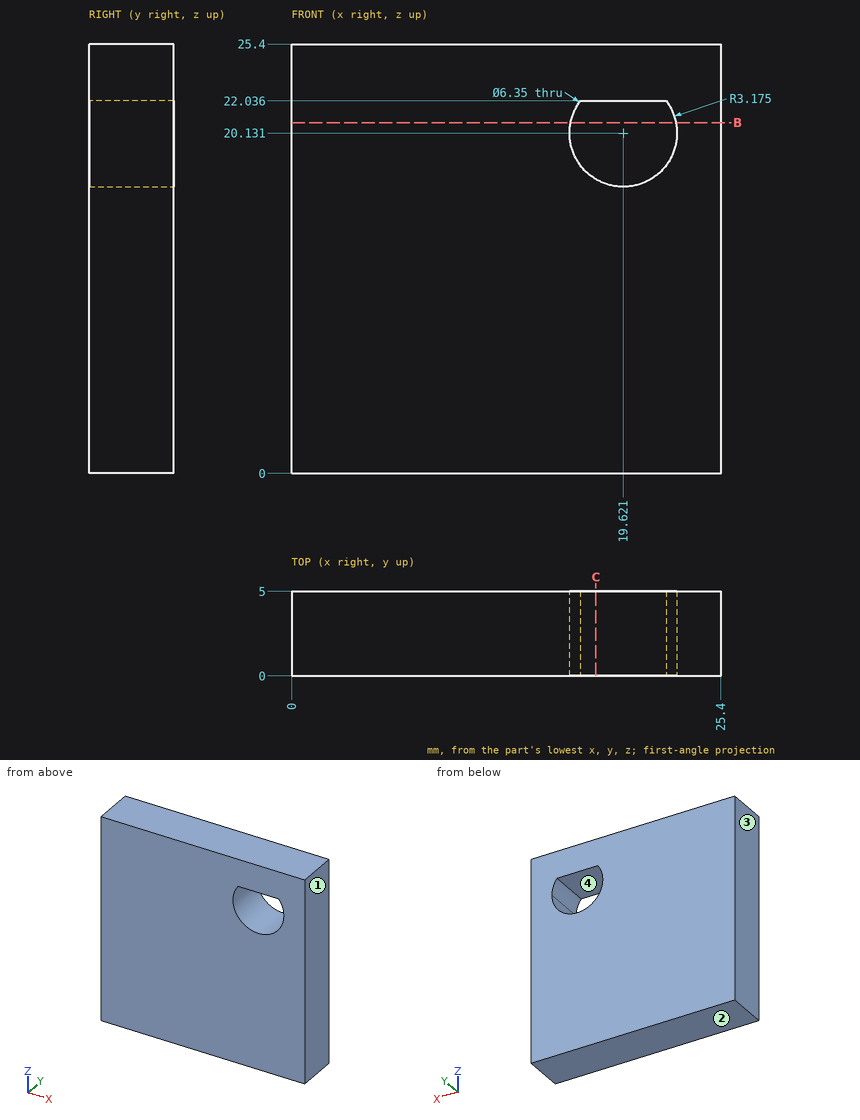
Drawing for the job (mm, zero at the part's lowest x, y, z). Give positions to 0.01 mm unless a question says otherwise; leave off trailing zeros. Order: outer loops, then holes, each group sorted by start corner. A loop starts at its lowest first (then second) coordinate and runs counter-clockwise, first axis right, second up. Notation, with made-up numbers: (-38, 64) - (17, 64) arc R19 ccw to (17, 69) - close; hole circle Ø3 at (58.5, -35.5). An arc over 180 degrees is marked (long way). Write item = value, one per line. Start each with the question number.
1. Cut at C-C, the plane x = 18. List the corners of the cut face in (y, z).
2. Cut at B-B, the plane z = 20.75. List the corners of the cut face in (x, y) (1 decimal).
3. Probe line 1 along Z through (x, y) = (19.5, 0.6); line 2 along Z through (x, y) = (17, 4.65) (1 decimal); line 3 along X through (y, z) = (4, 18.5) (1 decimal). List the from-to ranges inside material, lowest first.
4. Two-plate mould, pull along X, no slides. Class the marked faces 1, 2, 3 and 4: pulls with the +X half, pulls with the -X half, needs draft (parallel to the pull), parting line crosses it, or undercut.
Taken from the geometry:
q1.outline = (0, 0) - (5, 0) - (5, 17.4) - (0, 17.4) - close; (0, 22.04) - (5, 22.04) - (5, 25.4) - (0, 25.4) - close
q2.outline = (0, 0) - (16.5, 0) - (16.5, 5) - (0, 5) - close; (22.7, 0) - (25.4, 0) - (25.4, 5) - (22.7, 5) - close
q3.line_1 = 0 to 16.96, 22.04 to 25.4
q3.line_2 = 0 to 18.3, 21.9 to 25.4
q3.line_3 = 0 to 16.9, 22.3 to 25.4
q4.face_1 = pulls with the +X half
q4.face_2 = needs draft
q4.face_3 = pulls with the -X half
q4.face_4 = undercut
